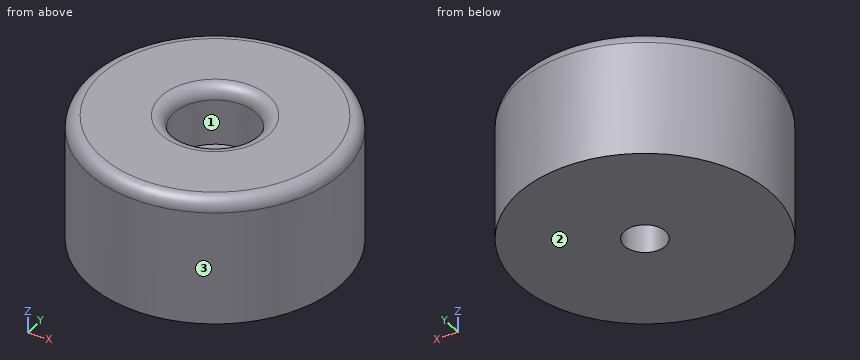
Autodesk Inventor part; units mm, degrees
ref_plane "YZ Plane" through (0, 0, 0) normal (1, 0, 0) x (0, 1, 0)
ref_plane "XZ Plane" through (0, 0, 0) normal (0, 1, 0) x (-1, 0, 0)
ref_plane "XY Plane" through (0, 0, 0) normal (0, 0, 1) x (1, 0, 0)
sketch "Sketch1" plane through (0, 0, 0) normal (0, 0, 1) x (1, 0, 0)
  circle A0 centre (0, 0) radius 20
  dimension "d0" = 40
extrude "Extrusion1" add sketch "Sketch1" along normal blind 20
sketch "Sketch2" plane through (0, 0, 20) normal (0, 0, 1) x (1, 0, 0)
  circle A0 centre (0, 0) radius 20
  circle A1 centre (0, 0) radius 6.5
  dimension "d4" = 13
extrude "Extrusion2" cut sketch "Sketch2" against normal blind 9.17 contours A1
sketch "Sketch3" plane through (0, 0, 10.83) normal (0, 0, 1) x (1, 0, 0)
  circle A0 centre (0, 0) radius 6.5
  circle A1 centre (0, 0) radius 3.25
  dimension "d8" = 6.5
extrude "Extrusion3" cut sketch "Sketch3" against normal through all contours A1
fillet "Fillet1" radius 2 2 edges at (-20, 0, 20) (-6.5, 0, 20)
properties part number "foot"
Geometry check sheet. Reference: the model listing, model coordinates, mm. Face numbers are marked on the shaded views. Round coordinates to 2 decimals unless told otherwise and drop trailing zeros. Order: outer loops, then holes, each group sorted by start corner. A loop starts at its lowest first (then second) coordinate and runs counter-clockwise, first axis right, second up. Notation, with made-up numbers: (73, 36.5) -> (122, 36.5) arc R19 ccw to (122, 55.5) -> close; hole circle Ø9 at (28, 12.25). An arc over 180 degrees is marked (long way). Return JSON: item names as keys, results as strings. Group by question number.
Q1. Gauge pin test, flat ends, axial feed: pin 1 (1.5 mm diameter, centred on y = 9, z = 18, fed in from -X); pin 2 (8 mm diameter, centred on y = 8.5, z = 14, fed in from -X); pin 3 (10.5 mm diameter, centred on x = 0, y = 0, fed in from +Z); pin 4 (8 mm diameter, centred on x = -3, y = 10.5, fed in from -Z). Record the tip position at first contact, or that the pin passes through.
Q2. Section check C-C, the plane z = 5.5. Record the boundary of the cut face in (x, y), plus the area to 3 significant figures.
Q3. Release check for a two-part mould opening along Y. For the marked faces 1, 2 and 3 record: released by +Y, released by -Y, zero draft, split by the parting line, or undercut.
Q4. Section check D-D, the plane z = 15.5. Record the boundary of the cut face in (x, y).
Q5. Material ranges on probe 1 along Y at (x, z) = (0, 14.75); probe 2 along Y at (x, z) = (0, 2.75); probe 3 along X at (y, z) = (1, 7.5), recorded low to high. Write a range as from..to.
Q6. Section check A-A, the plane y = 0. Record the boundary of the cut face in (x, z), plus the area to 3 significant figures.
Numbers:
{
 "1": {"pin 1": "x = -18.22", "pin 2": "x = -19.49", "pin 3": "z = 10.83", "pin 4": "z = 0"},
 "2": {"outline": "circle Ø40 at (0, 0); hole circle Ø6.5 at (0, 0)", "area": "1,220 mm^2"},
 "3": {"face 1": "undercut", "face 2": "zero draft", "face 3": "split by the parting line"},
 "4": {"outline": "circle Ø40 at (0, 0); hole circle Ø13 at (0, 0)"},
 "5": {"probe 1": "-20..-6.5, 6.5..20", "probe 2": "-20..-3.25, 3.25..20", "probe 3": "-19.97..-3.09, 3.09..19.97"},
 "6": {"outline": "(-20, 0) -> (-3.25, 0) -> (-3.25, 10.83) -> (-6.5, 10.83) -> (-6.5, 18) arc R2 ccw to (-8.5, 20) -> (-18, 20) arc R2 ccw to (-20, 18) -> close; (3.25, 0) -> (20, 0) -> (20, 18) arc R2 ccw to (18, 20) -> (8.5, 20) arc R2 ccw to (6.5, 18) -> (6.5, 10.83) -> (3.25, 10.83) -> close", "area": "607 mm^2"}
}
